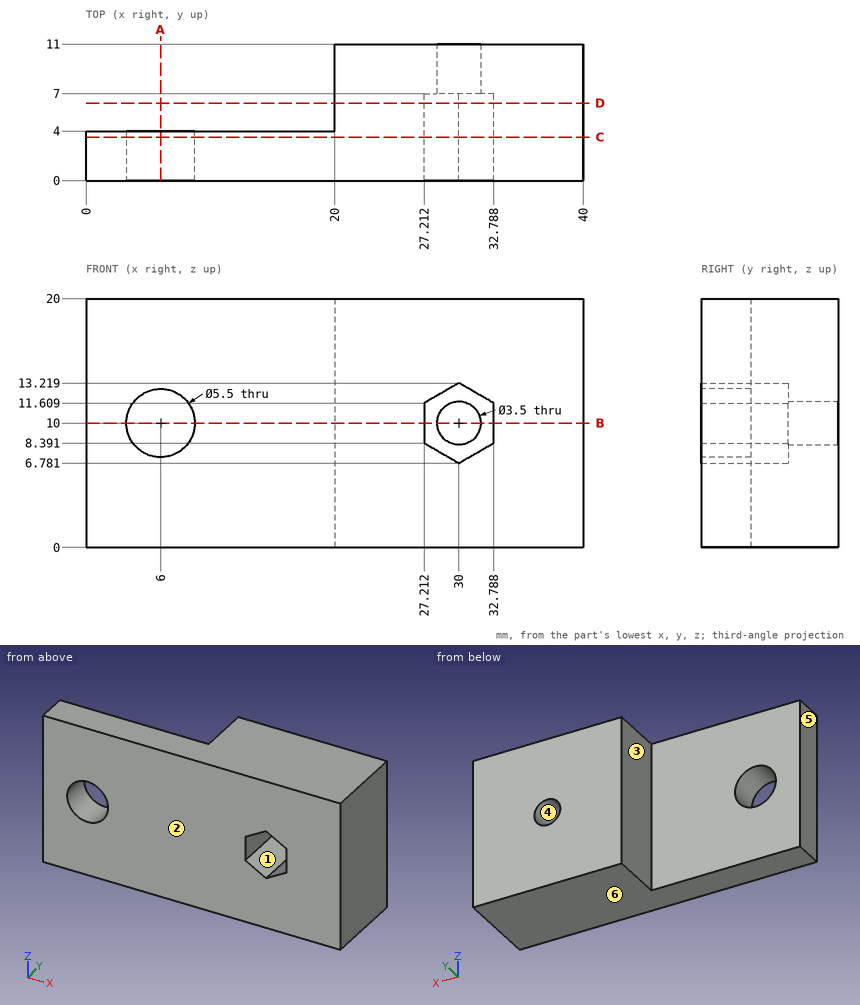
Here's the drawing with two shaded views (mm, measured from the low corner). I have some questions. A direction names the side the tool comes from. Give positions to 0.01 mm unless a question says otherwise; leave off trailing zeros. Write each loop counter-clockwise with the first axis right and the second up, starting at its lowest first coordinate (ties: lowest second). Pieces come first, ordered by that corner, then holes. Notation, with made-up numbers: (8.25, 9) -> (51.25, 9) arc R26 ccw to (51.25, 33) -> close; hole circle Ø1 at (85.25, 26). An arc over 180 degrees is marked (long way). Use one line per item in the form item = value. Start each with the question number.
1. Will these pins go through, and if not, where does the flat tip stop? pin 1 Ø2 at (y, z) = (8, 12) entering from -X; pin 2 Ø6.5 at (x, z) = (6, 10) entering from +Y; pin 3 Ø8 at (x, z) = (8.5, 14.5) entering from -Y; pin 4 Ø4 at (x, z) = (30, 10) entering from -Y.
2. If I drill on L1, parallel to X at y = 0.8, z = 10; L2, parallel to X at y = 9.8, z = 10; L3, parallel to Z at x = 6, y = 3.25, over which ranges is the centre line in solid material (lowest first)?
3. Imagine slicing it at C-C on y = 3.5. List the corners of the cut face in (x, z) for me, plus the area to 3 significant figures.
4. On a 3-axis mill with a long thin cutter (end or side, diameter ignored), from which of +Z, -Z, +X, -X, +Y, -Y can I reach the whole of each face in a straight line? I mean the marked faces 1, 2 and 3. Say none if no direction works.
5. Imagine slicing it at D-D on y = 6.25. List the corners of the cut face in (x, z) for me, plus the area to 3 significant figures.
6. Imagine slicing it at B-B on z = 10. List the corners of the cut face in (x, y) for me.
7. Imagine slicing it at A-A on x = 6. List the corners of the cut face in (y, z) for me, plus the area to 3 significant figures.
8. Thinking about a two-plate mould opening in X: for the marked faces 4, 5 and 6, which applies, +X half, -X half, draft (parallel to the pull), parting line (faces both ways), or undercut?
Entries:
q1.pin_1 = 20
q1.pin_2 = 4
q1.pin_3 = 0
q1.pin_4 = 7
q2.L1 = 0 to 3.25, 8.75 to 27.21, 32.79 to 40
q2.L2 = 20 to 28.25, 31.75 to 40
q2.L3 = 0 to 7.25, 12.75 to 20
q3.outline = (0, 0) -> (40, 0) -> (40, 20) -> (0, 20) -> close; hole circle Ø5.5 at (6, 10); hole (27.21, 8.39) -> (30, 6.78) -> (32.79, 8.39) -> (32.79, 11.61) -> (30, 13.22) -> (27.21, 11.61) -> close
q3.area = 749 mm²
q4.face_1 = -Y
q4.face_2 = +Z, -Z, +X, -X, -Y
q4.face_3 = +Z, -Z, -X, +Y
q5.outline = (20, 0) -> (40, 0) -> (40, 20) -> (20, 20) -> close; hole (27.21, 8.39) -> (30, 6.78) -> (32.79, 8.39) -> (32.79, 11.61) -> (30, 13.22) -> (27.21, 11.61) -> close
q5.area = 373 mm²
q6.outline = (0, 0) -> (3.25, 0) -> (3.25, 4) -> (0, 4) -> close; (8.75, 0) -> (27.21, 0) -> (27.21, 7) -> (28.25, 7) -> (28.25, 11) -> (20, 11) -> (20, 4) -> (8.75, 4) -> close; (31.75, 7) -> (32.79, 7) -> (32.79, 0) -> (40, 0) -> (40, 11) -> (31.75, 11) -> close
q7.outline = (0, 0) -> (4, 0) -> (4, 7.25) -> (0, 7.25) -> close; (0, 12.75) -> (4, 12.75) -> (4, 20) -> (0, 20) -> close
q7.area = 58.0 mm²
q8.face_4 = undercut
q8.face_5 = -X half
q8.face_6 = draft
